Geometry: final body of the model. Coordinates: model frame, mm. A direction names the side the tool comes from. Give positions to 0.01 mm unless a question says otherwise; leave off trailing zeros. Order: outer loops, then holes, each group sorted by start corner. A loop starts at its lowest first (then second) coordinate and runs counter-clockwise, first axis right, second up. Notation, with made-up numbers: (-12.5, 23.5) - (3.5, 23.5) arc R24 ccw to (3.5, 47.5) - close; hole circle Ø5 at (1, 77.5). An arc over 180 degrees is marked (long way). Use one line per item in the form item = value.
Autodesk Inventor part; units mm, degrees
ref_plane "YZ Plane" through (0, 0, 0) normal (1, 0, 0) x (0, 1, 0)
ref_plane "XZ Plane" through (0, 0, 0) normal (0, 1, 0) x (-1, 0, 0)
ref_plane "XY Plane" through (0, 0, 0) normal (0, 0, 1) x (1, 0, 0)
sketch "Sketch1" plane through (0, 0, 0) normal (1, 0, 0) x (0, 1, 0)
  circle A0 centre (-58.6732, 0) radius 31.02 construction
  line L0 (-39.6195, 0) -> (-14.1298, -32.6253) construction
  line L1 (-30.13, -12.146) -> (-30.13, 12.146) construction
  line L2 (0, 0) -> (-214.2426, 0) construction
  line L3 (-30.13, 12.146) -> (-33.107, -11.7755)
  line L4 (-33.107, -11.7755) -> (-30.13, -12.146)
  line L5 (-30.13, -12.146) -> (-27.153, 11.7755)
  line L6 (-27.153, 11.7755) -> (-30.13, 12.146)
  line L7 (-30.13, 12.146) -> (-30.13, -12.146) construction
  line L8 (-33.107, -11.7755) -> (-27.153, 11.7755) construction
  point P0 (-30.13, 0)
  dimension "d0" = 62.04
  dimension "d2" = 52
  dimension "d3" = 24.292
  dimension "d8" = 31.2206
  dimension "d9" = 16.0002
  dimension "d11" = 3
  dimension "d13" = 24.106
sketch "Sketch2" plane through (0, 0, 0) normal (1, 0, 0) x (0, 1, 0)
  line L0 (0, 0) -> (63.4666, 0)
  line L1 (63.4666, 0) -> (63.4666, -24.106)
  line L2 (63.4666, -24.106) -> (0, -24.106)
  line L3 (0, -24.106) -> (0, 0) construction
  line L4 (63.4666, -12.053) -> (-45.5912, -12.053) construction
  arc A0 (0, -24.106) -> (0, 0) centre (-28.5826, -12.053) ccw
  arc A1 (0, 0) -> (0, -24.106) centre (-28.5826, -12.053) ccw construction
  line L5 (80.4558, -9.553) -> (46.4774, -9.553) construction
  line L6 (46.4774, -9.553) -> (46.4774, -14.553) construction
  line L7 (46.4774, -14.553) -> (80.4558, -14.553) construction
  line L8 (80.4558, -14.553) -> (80.4558, -9.553) construction
  line L9 (80.4558, -9.553) -> (46.4774, -14.553) construction
  line L10 (46.4774, -9.553) -> (80.4558, -14.553) construction
  line L11 (43.4774, -9.553) -> (83.4558, -9.553)
  line L12 (83.4558, -9.553) -> (83.4558, -14.553) construction
  line L13 (83.4558, -14.553) -> (43.4774, -14.553)
  line L14 (43.4774, -14.553) -> (43.4774, -9.553)
  line L15 (43.4774, -9.553) -> (83.4558, -14.553) construction
  line L16 (83.4558, -9.553) -> (43.4774, -14.553) construction
  line L17 (78.4666, -26.1591) -> (48.4666, -26.1591)
  line L18 (48.4666, -26.1591) -> (48.4666, -22.053)
  line L19 (48.4666, -22.053) -> (78.4666, -22.053)
  line L20 (78.4666, -22.053) -> (78.4666, -26.1591)
  line L21 (78.4666, -26.1591) -> (48.4666, -22.053) construction
  line L22 (48.4666, -26.1591) -> (78.4666, -22.053) construction
  line L23 (48.4666, 2.053) -> (48.4666, -2.053)
  line L24 (48.4666, -2.053) -> (78.4666, -2.053)
  point P0 (63.4666, -9.553)
  point P1 (63.4666, -2.053)
  point P2 (48.4666, 0)
  point P3 (48.4666, -24.106)
  point P4 (63.4666, -22.053)
  point P5 (63.4666, -14.553)
  dimension "d12" = 24.106
  dimension "d14" = 62.04
  dimension "d15" = 63.4666
  dimension "d17" = 109.0578
  dimension "d18" = 44.04
  dimension "d19" = 5
  dimension "d20" = 3
  dimension "d22" = 30
  dimension "d25" = 20
extrude "Extrusion1" add sketch "Sketch2" along normal blind 3 contours L0 L23 L24 L1 L11 L14 L13 L19 L18 L2 A0
equation "\"d12\" = d13"
properties part number "Paleta" material "Laminate, Navy"
(1) Cut plane D-D on z = -10.5. Output: boundary loops of the cut face in (x, y), plus the area to 3 significant figures.
Computed values:
outline = (0, 2.4) - (3, 2.4) - (3, 43.48) - (0, 43.48) - close
area = 123 mm²
(2) Cut plane A-A on y = 50. Output: boundary loops of the cut face in (x, z), plus the area to 3 significant figures.
Computed values:
outline = (0, -22.05) - (3, -22.05) - (3, -14.55) - (0, -14.55) - close; (0, -9.55) - (3, -9.55) - (3, -2.05) - (0, -2.05) - close
area = 45.0 mm²
(3) Reachability of faces 4 (the face through (1, 48.467, -23)), 5 (the face through (1, 63.467, -6)), 6 (the face through (1, 24, 0)), 7 (the face through (1, 56, -2.053)), 8 (the face through (1, 53, -9.553)) from +Z, -Z, +X, -X, +Y, -Y: full face, straight path, thin tool, end or side. Return the list, or none.
Computed values:
face_4 = -Z, +X, -X, +Y
face_5 = +Z, -Z, +X, -X, +Y
face_6 = +Z, +X, -X, +Y, -Y
face_7 = +Z, +X, -X, +Y
face_8 = +X, -X, +Y
(4) Ray query, line 1 along Z through (x, y) = (2.3, 58); line 2 along Y through (x, z) = (2.5, -2.5); line 3 along Y through (x, z) = (0.25, -12.75). Return the intervals inside material, ascending.
Computed values:
line_1 = -22.05 to -14.55, -9.55 to -2.05
line_2 = 0.93 to 63.47
line_3 = 2.43 to 43.48
(5) Contact query for flat-ended pins moving along their axis: pin 1 Ø1 at (x, z) = (1.5, -1) entering from +Y; pin 2 Ø0.9 at (x, y) = (2, 58) entering from -Z; pin 3 Ø1.5 at (x, y) = (1, 50.5) entering from +Z. Output: stop coordinate, or through.
Computed values:
pin_1 = 48.47
pin_2 = -22.05
pin_3 = -2.05
(6) Cut plane B-B on x = 0.9. Output: boundary loops of the cut face in (y, z).
Computed values:
outline = (0, -24.11) - (48.47, -24.11) - (48.47, -22.05) - (63.47, -22.05) - (63.47, -14.55) - (43.48, -14.55) - (43.48, -9.55) - (63.47, -9.55) - (63.47, -2.05) - (48.47, -2.05) - (48.47, 0) - (0, 0) arc R31.02 cw to start
(7) Pull-direction query (Z, two-part tool) for faces 1 (the face through (1.479, 2.437, -11.88)), 2 (the face through (1, 63.467, -18)), 3 (the face through (1, 25, -24.106)); classes: released by +Z, released by -Z, zero draft, split by the parting line, or undercut.
Computed values:
face_1 = undercut
face_2 = zero draft
face_3 = released by -Z
(8) Cut plane C-C on z = -6.75. Output: boundary loops of the cut face in (x, y), plus the area to 3 significant figures.
Computed values:
outline = (0, 1.98) - (3, 1.98) - (3, 63.47) - (0, 63.47) - close
area = 184 mm²
